```python
from build123d import *

# Parameters (mm, degrees)
BOSS_EXTRUDE1_DEPTH = 35
SKETCH2_R           = 12.75
CUT_EXTRUDE1_DEPTH  = 32
CUT_EXTRUDE2_REACH  = 37
SKETCH3_R           = 1.5
SKETCH3_R_2         = 3.75
CUT_EXTRUDE3_REACH  = 7
SKETCH4_R           = 3.2
FILLET1_R           = 2
FILLET3_R           = 6
FILLET4_R           = 6


with BuildPart() as part:
    # Sketch1 → Boss-Extrude1 (new body)
    with BuildSketch(Plane(origin=(0, 0, 0), x_dir=(0, 0, -1), z_dir=(1, 0, 0))):
        with BuildLine():
            Line((-48, -55), (-48, -50))
            Line((-48, -50), (-20, -50))
            Line((-20, -50), (-20, 0))
            ThreePointArc((-20, 0), (0, 20), (20, 0))
            Line((20, 0), (20, -50))
            Line((20, -50), (48, -50))
            Line((48, -50), (48, -55))
            Line((48, -55), (-48, -55))
        make_face()
    extrude(amount=BOSS_EXTRUDE1_DEPTH)

    # Sketch2 → Cut-Extrude1 (cut)
    with BuildSketch(Plane(origin=(35, 0, 0), x_dir=(0, 0, -1), z_dir=(1, 0, 0))):
        Circle(SKETCH2_R)
    extrude(amount=-CUT_EXTRUDE1_DEPTH, mode=Mode.SUBTRACT)

    # Sketch3 → Cut-Extrude2 (cut, up to next)
    with BuildSketch(Plane.ZY, mode=Mode.PRIVATE) as cut_extrude2_sk1:
        with Locations((0, 8.5)):
            Circle(SKETCH3_R)
    cut_extrude2_tool1 = extrude(cut_extrude2_sk1.sketch, amount=-CUT_EXTRUDE2_REACH, mode=Mode.PRIVATE) & part.part
    add(cut_extrude2_tool1.solids().sort_by_distance((0, 8.5, 0))[0], mode=Mode.SUBTRACT)
    # Sketch3 → Cut-Extrude2 (cut, up to next)
    with BuildSketch(Plane.ZY, mode=Mode.PRIVATE) as cut_extrude2_sk2:
        with Locations((0, -8.5)):
            Circle(SKETCH3_R)
    cut_extrude2_tool2 = extrude(cut_extrude2_sk2.sketch, amount=-CUT_EXTRUDE2_REACH, mode=Mode.PRIVATE) & part.part
    add(cut_extrude2_tool2.solids().sort_by_distance((0, -8.5, 0))[0], mode=Mode.SUBTRACT)
    # Sketch3 → Cut-Extrude2 (cut, up to next)
    with BuildSketch(Plane.ZY, mode=Mode.PRIVATE) as cut_extrude2_sk3:
        Circle(SKETCH3_R_2)
    cut_extrude2_tool3 = extrude(cut_extrude2_sk3.sketch, amount=-CUT_EXTRUDE2_REACH, mode=Mode.PRIVATE) & part.part
    add(cut_extrude2_tool3.solids().sort_by_distance((0, 0, 0))[0], mode=Mode.SUBTRACT)

    # Sketch4 → Cut-Extrude3 (cut, up to next)
    with BuildSketch(Plane(origin=(0, -50, 0), x_dir=(1, 0, 0), z_dir=(0, 1, 0)), mode=Mode.PRIVATE) as cut_extrude3_sk1:
        with Locations((17.5, 37.5)):
            Circle(SKETCH4_R)
    cut_extrude3_tool1 = extrude(cut_extrude3_sk1.sketch, amount=-CUT_EXTRUDE3_REACH, mode=Mode.PRIVATE) & part.part
    add(cut_extrude3_tool1.solids().sort_by_distance((17.5, -50, -37.5))[0], mode=Mode.SUBTRACT)
    # Sketch4 → Cut-Extrude3 (cut, up to next)
    with BuildSketch(Plane(origin=(0, -50, 0), x_dir=(1, 0, 0), z_dir=(0, 1, 0)), mode=Mode.PRIVATE) as cut_extrude3_sk2:
        with Locations((17.5, -37.5)):
            Circle(SKETCH4_R)
    cut_extrude3_tool2 = extrude(cut_extrude3_sk2.sketch, amount=-CUT_EXTRUDE3_REACH, mode=Mode.PRIVATE) & part.part
    add(cut_extrude3_tool2.solids().sort_by_distance((17.5, -50, 37.5))[0], mode=Mode.SUBTRACT)

    # Fillet1
    fillet1_edges = [part.edges().sort_by_distance(p)[0] for p in [
        (35, 0, 12.75),
    ]]
    fillet(fillet1_edges, radius=FILLET1_R)

    # Fillet3
    fillet3_edges = [part.edges().sort_by_distance(p)[0] for p in [
        (17.5, -50, 20),
        (17.5, -50, -20),
    ]]
    fillet(fillet3_edges, radius=FILLET3_R)

    # Fillet4
    fillet4_edges = [part.edges().sort_by_distance(p)[0] for p in [
        (0, -52.5, -48),
        (35, -52.5, 48),
        (0, -52.5, 48),
        (35, -52.5, -48),
    ]]
    fillet(fillet4_edges, radius=FILLET4_R)


solid = part.part
```
Can you work these out from the model? Positions are in its coordinate system, mm. A direction names the side the tool comes from. Coordinates: 2 decimals unless noted, no trailing zeros. Write each loop counter-clockwise with the first axis right and the second up, starting at its lowest first coordinate (ties: lowest second). Pieces come first, ordered by that corner, then holes. Notation, with made-up numbers: M -27,42 L 18,42 A11 cw 18,52 Z; hole C -29,70 d5. An arc over 180 degrees is marked long. Answer as CSV lines item,"result".
Item 1: Please list where these lines run through material, in increasing order: line 1 along Z through (x, y) = (17.5, -53.4); line 2 along Y through (x, z) = (21.5, 0); line 3 along Y through (x, z) = (1, 0).
Geometry results:
line 1,"z = -48 to -40.7, -34.3 to 34.3, 40.7 to 48"
line 2,"y = -55 to -12.75, 12.75 to 20"
line 3,"y = -55 to -10, -7 to -3.75, 3.75 to 7, 10 to 20"
Item 2: Imagine slicing it at C-C on x = 23. List the corners of the cut face in (y, z) for me.
Geometry results:
outline,"M -55,-48 L -50,-48 L -50,-26 A6 cw -44,-20 L 0,-20 A20 ccw 0,20 L -44,20 A6 cw -50,26 L -50,48 L -55,48 Z; hole C 0,0 d25.5"
Item 3: Imagine slicing it at D-D on z = 37.5. List the corners of the cut face in (x, y) for me, plus the area to 3 significant figures.
Geometry results:
outline,"M 0,-55 L 14.3,-55 L 14.3,-50 L 0,-50 Z; M 20.7,-55 L 35,-55 L 35,-50 L 20.7,-50 Z"
area,"143 mm2"
Item 4: Imagine slicing it at B-B on z = 0. List the corners of the cut face in (x, y) for me.
Geometry results:
outline,"M 0,-55 L 35,-55 L 35,-14.75 A2 ccw 33,-12.75 L 3,-12.75 L 3,-10 L 0,-10 Z; M 0,-7 L 3,-7 L 3,-3.75 L 0,-3.75 Z; M 0,3.75 L 3,3.75 L 3,7 L 0,7 Z; M 0,10 L 3,10 L 3,12.75 L 33,12.75 A2 ccw 35,14.75 L 35,20 L 0,20 Z"
Item 5: On a 3-axis mill with a long thin cutter (end or side, diameter ignored), from which of +Z, -Z, +X, -X, +Y, -Y can I reach the whole of each face in a straight line? I mean faces 4 (the cylindrical face through (18.21, -12.447, 2.764)), 5 (the flat face through (17, -22, 20)), 6 (the flat face through (21, -50, -37)), 7 (the cylindrical face through (1, -10, 0)), 8 (the cylindrical face through (33.289, -52.535, -46.196)). Say none if no direction works.
Geometry results:
face 4,"+X"
face 5,"+Z, +X, -X, +Y"
face 6,"-Z, +X, -X, +Y"
face 7,"+X, -X"
face 8,"-Z, +X, +Y, -Y"
Item 6: We'd pull the mould along Y, two halves only. Please class faces 1 (the flat face through (17, -55, -1)), 2 (the flat face through (17, -52, -48)), 3 (the flat face through (3, -3, -3)): +Y half, -Y half, draft (parallel to the pull), parting line (faces both ways), or undercut.
Geometry results:
face 1,"-Y half"
face 2,"draft"
face 3,"undercut"
Item 7: I'm going to push flat-ended pins straight in: P1, Ø8, axis at x = 22.5, y = -20, coming from the +Z side; P2, Ø8.5, axis at x = 17.5, z = 37.5, coming from the +Y side; P3, Ø3.5, axis at y = 8.5, z = 0, coming from the +X side. Where does each tip first touch, or does it pass through?
Geometry results:
P1,"stops at z = 20"
P2,"stops at y = -50"
P3,"stops at x = 3"
Item 8: Imagine slicing it at A-A on x = 17.5. List the corners of the cut face in (y, z) for me.
Geometry results:
outline,"M -55,-48 L -50,-48 L -50,-40.7 L -55,-40.7 Z; M -55,-34.3 L -50,-34.3 L -50,-26 A6 cw -44,-20 L 0,-20 A20 ccw 0,20 L -44,20 A6 cw -50,26 L -50,34.3 L -55,34.3 Z; M -55,40.7 L -50,40.7 L -50,48 L -55,48 Z; hole C 0,0 d25.5"
